from build123d import *

# Parameters (mm, degrees)
F0_W     = 19.05
F0_H     = 50.8
F0_W_2   = 152.4
F0_H_2   = 19.05
F0_H_3   = 19.0500013826
F1_DEPTH = 19.05


# Not quite as in the source:
# - a feature names something its author has since deleted; it is built from what else it names


with BuildPart() as f1:
    # F0 (on Front) → F1 (new body)
    with BuildSketch(Plane.XZ):
        Polygon((-511.175, 0), (-739.775, 0), (-739.775, -514.35), (-511.175, -514.35), (-358.775, -514.35), (358.775, -514.35), (511.175, -514.35), (739.775, -514.35), (739.775, 0), (511.175, 0), (358.775, 0), (-358.775, 0), align=None)
        with Locations((-243.4166649733, -457.2)):
            Rectangle(F0_W, F0_H, mode=Mode.SUBTRACT)
        with Locations((-365.125, -390.525)):
            Rectangle(F0_W_2, F0_H_2, mode=Mode.SUBTRACT)
        with Locations((-243.4166666497, -323.85)):
            Rectangle(F0_W, F0_H, mode=Mode.SUBTRACT)
        with Locations((-365.125, -257.175)):
            Rectangle(F0_W_2, F0_H_2, mode=Mode.SUBTRACT)
        with Locations((243.41666836, -457.2000013826)):
            Rectangle(F0_W, F0_H, mode=Mode.SUBTRACT)
        with Locations((365.125, -390.5250006913)):
            Rectangle(F0_W_2, F0_H_3, mode=Mode.SUBTRACT)
        with Locations((243.4166666836, -323.85)):
            Rectangle(F0_W, F0_H, mode=Mode.SUBTRACT)
        with Locations((365.125, -257.175)):
            Rectangle(F0_W_2, F0_H_2, mode=Mode.SUBTRACT)
        with Locations((-243.416666665, -190.5)):
            Rectangle(F0_W, F0_H, mode=Mode.SUBTRACT)
        with Locations((-365.125, -123.825)):
            Rectangle(F0_W_2, F0_H_2, mode=Mode.SUBTRACT)
        with Locations((-243.416666665, -57.15)):
            Rectangle(F0_W, F0_H, mode=Mode.SUBTRACT)
        with Locations((243.4166666684, -190.5)):
            Rectangle(F0_W, F0_H, mode=Mode.SUBTRACT)
        with Locations((365.125, -123.825)):
            Rectangle(F0_W_2, F0_H_2, mode=Mode.SUBTRACT)
        with Locations((243.4166666684, -57.15)):
            Rectangle(F0_W, F0_H, mode=Mode.SUBTRACT)
        with Locations((-434.975, 9.525)):
            Rectangle(F0_W_2, F0_H_2)
        with Locations((434.975, 9.525)):
            Rectangle(F0_W_2, F0_H_2)
        with Locations((-434.975, -523.875)):
            Rectangle(F0_W_2, F0_H_2)
        with Locations((434.975, -523.875)):
            Rectangle(F0_W_2, F0_H_2)
    extrude(amount=F1_DEPTH)


solid = f1.part
Could you check a few things on this model? Use its own coordinates, in mm. Coordinates: 2 decimals unless noted, no trailing zeros. Order: outer loops, then holes, each group sorted by start corner. A loop starts at its lowest first (then second) coordinate and runs counter-clockwise, first axis right, second up. Notation, with made-up numbers: (-17, 2.5) -> (-10, 2.5) arc R16 ccw to (-10, 17.5) -> close; hole circle Ø6 at (68.5, -20). An arc over 180 degrees is marked (long way). One line per item, written item: value. Start each with the question number.
1) Imagine slicing it at C-C on y = -3. Count the separate pieces of the cut face and the enclosed holes in it, plus the area to 3 significant figures.
2) Imagine slicing it at D-D on x = 547.5. List the corners of the cut face in (y, z) for me, plus the area to 3 significant figures.
3) Imagine slicing it at B-B on z = -201. List the corners of the cut face in (x, y) for me (3 decimals), plus the area to 3 significant figures.
4) If I drill on L1, parallel to X at y = -16.75, z = -250.5 (3 decimals); L2, parallel to X at y = -17, z = -315.5 (3 decimals); L3, parallel to Z at x = -390, y = -16, over which ranges is the centre line in solid material (lowest first)? Write a range as [from, to].
5) Imagine slicing it at A-A on x = 319.5. List the corners of the cut face in (y, z) for me.
6) I'm going to push flat-ended pins straight in: pin 1 (9.5 mm diameter, centred on y = -9.5, z = -524, fed in from -X) (3 decimals); pin 2 (1 mm diameter, centred on x = -0.5, y = -8.5, fed in from -Z); pin 3 (6 mm diameter, centred on x = 34.5, y = -7, fed in from +Z). Where does each tip first touch, or does it pass through?
Answer list:
1. separate pieces: 1
1. enclosed holes: 14
1. area: 747,000 mm2
2. outline: (-19.05, -514.35) -> (0, -514.35) -> (0, 0) -> (-19.05, 0) -> close
2. area: 9,800 mm2
3. outline: (-739.775, -19.05) -> (-252.942, -19.05) -> (-252.942, 0) -> (-739.775, 0) -> close; (-233.892, -19.05) -> (233.892, -19.05) -> (233.892, 0) -> (-233.892, 0) -> close; (252.942, -19.05) -> (739.775, -19.05) -> (739.775, 0) -> (252.942, 0) -> close
3. area: 27,500 mm2
4. L1: x = [-739.775, -441.325], [-288.925, 288.925], [441.325, 739.775]
4. L2: x = [-739.775, -252.942], [-233.892, 233.892], [252.942, 739.775]
4. L3: z = [-533.4, -400.05], [-381, -266.7], [-247.65, -133.35], [-114.3, 19.05]
5. outline: (-19.05, -514.35) -> (0, -514.35) -> (0, -400.05) -> (-19.05, -400.05) -> close; (-19.05, -381) -> (0, -381) -> (0, -266.7) -> (-19.05, -266.7) -> close; (-19.05, -247.65) -> (0, -247.65) -> (0, -133.35) -> (-19.05, -133.35) -> close; (-19.05, -114.3) -> (0, -114.3) -> (0, 0) -> (-19.05, 0) -> close
6. pin 1: stops at x = -511.175
6. pin 2: stops at z = -514.35
6. pin 3: stops at z = 0
